from build123d import *

# Parameters (mm, degrees)
SKETCH1_R           = 7.25
BOSS_EXTRUDE1_DEPTH = 1
SKETCH2_R           = 5.5
BOSS_EXTRUDE2_DEPTH = 3
SKETCH3_R           = 9.5
BOSS_EXTRUDE3_DEPTH = 1.2
SKETCH4_R           = 9.5
SKETCH4_R_2         = 5.5
BOSS_EXTRUDE4_DEPTH = 4.5
SKETCH5_R           = 9.5
SKETCH5_R_2         = 8.1
BOSS_EXTRUDE5_DEPTH = 5


with BuildPart() as part:
    # Sketch1 → Boss-Extrude1 (new body)
    with BuildSketch(Plane(origin=(0, 0, 0), x_dir=(1, 0, 0), z_dir=(0, 1, 0))):
        with Locations(Location((0, 0, 0), (0, 0, 270))):
            Circle(SKETCH1_R)
    extrude(amount=BOSS_EXTRUDE1_DEPTH)

    # Sketch2 → Boss-Extrude2 (add)
    with BuildSketch(Plane(origin=(0, 1, 0), x_dir=(1, 0, 0), z_dir=(0, 1, 0))):
        with Locations(Location((0, 0, 0), (0, 0, 270))):
            Circle(SKETCH2_R)
    extrude(amount=BOSS_EXTRUDE2_DEPTH)

    # Sketch3 → Boss-Extrude3 (add)
    with BuildSketch(Plane(origin=(0, 4, 0), x_dir=(1, 0, 0), z_dir=(0, 1, 0))):
        with Locations(Location((0, 0, 0), (0, 0, 270))):
            Circle(SKETCH3_R)
    extrude(amount=BOSS_EXTRUDE3_DEPTH)

    # Sketch4 → Boss-Extrude4 (add)
    with BuildSketch(Plane(origin=(0, 5.2, 0), x_dir=(1, 0, 0), z_dir=(0, 1, 0))):
        with Locations(Location((0, 0, 0), (0, 0, 270))):
            Circle(SKETCH4_R)
        with Locations(Location((0, 0, 0), (0, 0, 270))):
            Circle(SKETCH4_R_2, mode=Mode.SUBTRACT)
    extrude(amount=BOSS_EXTRUDE4_DEPTH)

    # Sketch5 → Boss-Extrude5 (add)
    with BuildSketch(Plane(origin=(0, 9.7, 0), x_dir=(1, 0, 0), z_dir=(0, 1, 0))):
        with Locations(Location((0, 0, 0), (0, 0, 270))):
            Circle(SKETCH5_R)
        with Locations(Location((0, 0, 0), (0, 0, 270))):
            Circle(SKETCH5_R_2, mode=Mode.SUBTRACT)
    extrude(amount=BOSS_EXTRUDE5_DEPTH)


solid = part.part
Geometry: final body of the model. Coordinates: model frame, mm. A direction names the side the tool comes from. Give positions to 0.01 mm unless a question says otherwise; leave off trailing zeros. Write each loop counter-clockwise with the first axis right and the second up, starting at its lowest first coordinate (ties: lowest second). Pieces come first, ordered by that corner, then holes. Notation, with made-up numbers: (47, 11) -> (70, 11) arc R27 ccw to (70, 30) -> close; hole circle Ø6 at (-18.5, -4.5). An arc over 180 degrees is marked (long way). Answer as a JSON object with one key per item and string values.
1. Cut plane B-B on z = 0. Output: boundary loops of the cut face in (x, y), and give its area (3 significant figures).
Ans:
{"outline": "(-9.5, 4) -> (-5.5, 4) -> (-5.5, 1) -> (-7.25, 1) -> (-7.25, 0) -> (7.25, 0) -> (7.25, 1) -> (5.5, 1) -> (5.5, 4) -> (9.5, 4) -> (9.5, 14.7) -> (8.1, 14.7) -> (8.1, 9.7) -> (5.5, 9.7) -> (5.5, 5.2) -> (-5.5, 5.2) -> (-5.5, 9.7) -> (-8.1, 9.7) -> (-8.1, 14.7) -> (-9.5, 14.7) -> close", "area": "120 mm^2"}
2. Cut plane D-D on y = 3.25. Output: boundary loops of the cut face in (x, z), and give its area (3 significant figures).
Ans:
{"outline": "circle Ø11 at (0, 0)", "area": "95.0 mm^2"}
3. Mould query, pull axis Y, two halves, no side actions, for faces 1 (the flat face through (5, 1, 3)), 2 (the flat face through (0, 0, 0)), 3 (the cylindrical face through (-5.37, 2.48, -1.19)), 4 (the cylindrical face through (-7.186, 12.165, 3.738)). Classes: pulls with the +Y half, pulls with the -Y half, needs draft (parallel to the pull), parting line crosses it, or undercut.
Ans:
{"face 1": "undercut", "face 2": "pulls with the -Y half", "face 3": "undercut", "face 4": "needs draft"}
4. Contact query for flat-ended pins moving along their axis: pin 1 (9 mm diameter, centred on x = -1.5, z = -2, fed in from +Y); pin 2 (6 mm diameter, centred on x = 4, y = 13, fed in from +Z); pin 3 (1 mm diameter, centred on y = 12.5, z = -5, fed in from -X). Output: stop coordinate, or through.
Ans:
{"pin 1": "stops at y = 9.7", "pin 2": "stops at z = 9.45", "pin 3": "stops at x = -8.37"}
5. Cut plane C-C on x = 0. Output: boundary loops of the cut face in (y, z).
Ans:
{"outline": "(0, -7.25) -> (1, -7.25) -> (1, -5.5) -> (4, -5.5) -> (4, -9.5) -> (14.7, -9.5) -> (14.7, -8.1) -> (9.7, -8.1) -> (9.7, -5.5) -> (5.2, -5.5) -> (5.2, 5.5) -> (9.7, 5.5) -> (9.7, 8.1) -> (14.7, 8.1) -> (14.7, 9.5) -> (4, 9.5) -> (4, 5.5) -> (1, 5.5) -> (1, 7.25) -> (0, 7.25) -> close"}
6. Access query for faces 5 (the flat face through (6, 9.7, 0)), 6 (the flat face through (-4, 4, 4)), 7 (the cylindrical face through (-2.777, 0.493, 6.697)), 8 (the flat face through (3, 14.7, 8)), 9 (the cylindrical face through (-5.78, 9.28, -7.54)). Directions: +Z, -Z, +X, -X, +Y, -Y. A direction counts if a zero-diameter tool reaches every point of the face in a straight line with its end or side. Return the directions, or none.
Ans:
{"face 5": "+Y", "face 6": "none", "face 7": "-Y", "face 8": "+Z, -Z, +X, -X, +Y", "face 9": "+Y, -Y"}
7. Cut plane A-A on x = 5.75. Output: boundary loops of the cut face in (y, z).
Ans:
{"outline": "(0, -4.42) -> (1, -4.42) -> (1, 4.42) -> (0, 4.42) -> close; (4, -7.56) -> (14.7, -7.56) -> (14.7, -5.71) -> (9.7, -5.71) -> (9.7, 5.71) -> (14.7, 5.71) -> (14.7, 7.56) -> (4, 7.56) -> close"}
8. Ray query, probe 1 along X at (y, z) = (11.25, 0); probe 2 along Y at (x, z) = (-5.75, 1); probe 3 along X at (y, z) = (8, 0). Return the intervals inside material, ascending. Write a range as from..to.
Ans:
{"probe 1": "x = -9.5..-8.1, 8.1..9.5", "probe 2": "y = 0..1, 4..9.7", "probe 3": "x = -9.5..-5.5, 5.5..9.5"}
